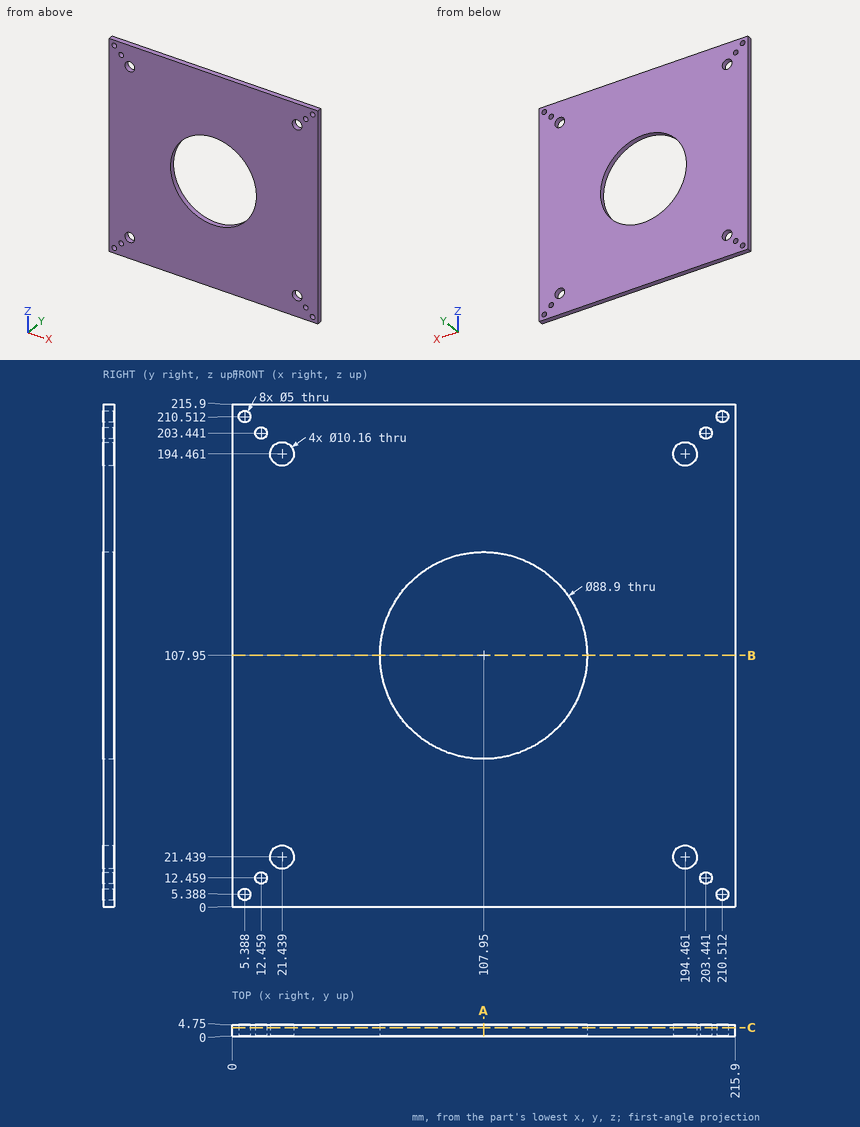
Design review of the part shown in the three views and the two pictorial views. Dimensions are in mm from the part's minimum x, y and z. Coordinates: 2 decimals unless noted, no trailing zeros. Write each loop counter-clockwise with the first axis right and the second up, starting at its lowest first coordinate (ties: lowest second). Pieces come first, ordered by that corner, then holes.
(1) Add section B-B on z = 107.95. Give the boundary of the cut face in (x, y).
(2) Add section C-C on y = 3.6. Count the separate pieces of the cut face and the enclosed holes in it, then the cut area to 3 significant figures.
(3) For pin 1 Ø9 at (x, z) = (21.44, 194.46) entering from -Y, flat-tipped, find the tip position at first contact; note if it passes through.
(4) Wall thickness on probe 1 along X at (y, z) = (0.6, 12.5); probe 2 along X at (y, z) = (0.2, 20.5); probe 3 along X at (y, z) = (1.95, 135): over which ranges is each line inside the solid? List them lowest first.
(5) Add section A-A on x = 107.95. Give the boundary of the cut face in (y, z).
Answer sheet:
1. outline: (0, 0) - (63.5, 0) - (63.5, 4.75) - (0, 4.75) - close; (152.4, 0) - (215.9, 0) - (215.9, 4.75) - (152.4, 4.75) - close
2. separate pieces: 1
2. enclosed holes: 13
2. area: 39,900 mm2
3. pin 1: passes through
4. probe 1: x = 0 to 9.96, 14.96 to 200.94, 205.94 to 215.9
4. probe 2: x = 0 to 16.45, 26.43 to 189.47, 199.45 to 215.9
4. probe 3: x = 0 to 72.68, 143.22 to 215.9
5. outline: (0, 0) - (4.75, 0) - (4.75, 63.5) - (0, 63.5) - close; (0, 152.4) - (4.75, 152.4) - (4.75, 215.9) - (0, 215.9) - close
